Can you work these out from the model? Positions are in its coordinate system, mm. Face numbers are marked on the shaded views. A direction names the side the tool comes from. Give positions to 0.01 mm unless a question says otherwise; leave off trailing zeros. Loops run counter-clockwise (first coordinate to the right, second up) from the corner with the lowest first, then second, coordinate; pieces in that order, holes last. Notation, with made-up numbers: (73, 34) - (102, 34) arc R22 ccw to (102, 52) - close; hole circle Ø10 at (-14.75, -37). An arc over 180 degrees is marked (long way). Answer as a JSON object with one key per item and string values.
```python
from build123d import *

# Parameters (mm, degrees)
ESQUISSE1_W        = 198.661449586
ESQUISSE1_H        = 145.541105456
BOSS_EXTRU_1_DEPTH = 20
ESQUISSE2_W        = 72.740275378
ESQUISSE2_H        = 59.392258424
BOSS_EXTRU_2_DEPTH = 60
CONG_1_R           = 5
CHANFREIN1_SIZE    = 10


with BuildPart() as part:
    # Esquisse1 → Boss.-Extru.1 (new body)
    with BuildSketch(Plane(origin=(0, 0, 0), x_dir=(1, 0, 0), z_dir=(0, 1, 0))):
        Rectangle(ESQUISSE1_W, ESQUISSE1_H)
    extrude(amount=BOSS_EXTRU_1_DEPTH)

    # Esquisse2 → Boss.-Extru.2 (add)
    with BuildSketch(Plane(origin=(0, 20, 0), x_dir=(1, 0, 0), z_dir=(0, 1, 0))):
        Rectangle(ESQUISSE2_W, ESQUISSE2_H)
    extrude(amount=BOSS_EXTRU_2_DEPTH)

    # Congé1
    cong_1_edges = [part.edges().sort_by_distance(p)[0] for p in [
        (36.370137689, 20, 0),
        (0, 20, -29.696129212),
        (-36.370137689, 20, 0),
        (0, 20, 29.696129212),
    ]]
    fillet(cong_1_edges, radius=CONG_1_R)

    # Chanfrein1
    chanfrein1_edges = [part.edges().sort_by_distance(p)[0] for p in [
        (99.330724793, 10, 72.770552728),
        (-99.330724793, 10, 72.770552728),
        (-99.330724793, 10, -72.770552728),
        (99.330724793, 10, -72.770552728),
    ]]
    chamfer(chanfrein1_edges, length=CHANFREIN1_SIZE)


solid = part.part
```
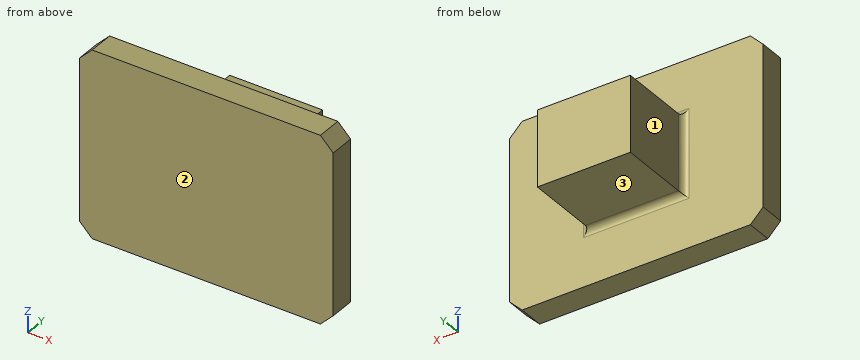
1) Which directions (+Z, -Z, +X, -X, +Y, -Y) give clear straight access to the entire face, cutting with the end or side of a thin tool? Please do the marked faces 1, 2 and 3.
Check sheet entries:
{"face 1": "+Z, -Z, -X, +Y", "face 2": "+Z, -Z, +X, -X, -Y", "face 3": "-Z, +X, -X, +Y"}
2) Imagine slicing it at D-D on x = -55.5. Write out the boundary of the cut face in (y, z), and give its area (3 significant figures).
Check sheet entries:
{"outline": "(0, -72.77) - (20, -72.77) - (20, 72.77) - (0, 72.77) - close", "area": "2,910 mm2"}
3) I need wall thicknesses on L1, parallel to X at y = 25.5, z = 28.5; L2, parallel to Y at x = -17, z = -63.5; L3, parallel to Z at x = -19, y = 39. Which ranges of each line are inside material? Lowest first, please.
Check sheet entries:
{"L1": "-36.37 to 36.37", "L2": "0 to 20", "L3": "-29.7 to 29.7"}
4) Imagine slicing it at B-B on x = 14. Write out the boundary of the cut face in (y, z).
Check sheet entries:
{"outline": "(0, -72.77) - (20, -72.77) - (20, -34.7) arc R5 cw to (25, -29.7) - (80, -29.7) - (80, 29.7) - (25, 29.7) arc R5 cw to (20, 34.7) - (20, 72.77) - (0, 72.77) - close"}
5) I'm going to push flat-ended pins straight in: P1, Ø6, axis at x = 64.5, z = -50.5, coming from the -Y side; P2, Ø6, axis at x = -21.5, y = 33.5, coming from the +Z side; P3, Ø16.5, axis at y = 64.5, z = -3, coming from the -X side; P4, Ø2, axis at x = -29, y = 69.5, coming from the -Z side. Where does each tip first touch, or does it pass through?
Check sheet entries:
{"P1": "y = 0", "P2": "z = 29.7", "P3": "x = -36.37", "P4": "z = -29.7"}
6) Imagine slicing it at C-C on y = 68. Write out the boundary of the cut face in (x, z), and give its area (3 significant figures).
Check sheet entries:
{"outline": "(-36.37, -29.7) - (36.37, -29.7) - (36.37, 29.7) - (-36.37, 29.7) - close", "area": "4,320 mm2"}
7) Imagine slicing it at A-A on z = -26. Write out the boundary of the cut face in (x, y), and give its area (3 significant figures).
Check sheet entries:
{"outline": "(-99.33, 0) - (99.33, 0) - (99.33, 20) - (41.37, 20) arc R5 cw to (36.37, 25) - (36.37, 80) - (-36.37, 80) - (-36.37, 25) arc R5 cw to (-41.37, 20) - (-99.33, 20) - close", "area": "8,350 mm2"}
